Design review of the part built by this model. Coordinates are the model's own, in mm. A direction names the side the tool comes from. Coordinates: 2 decimals unless noted, no trailing zeros. Loops run counter-clockwise (first coordinate to the right, second up) from the corner with the lowest first, then second, coordinate; pieces in that order, holes last. Notation, with made-up numbers: (65.25, 86.25) -> (108.25, 86.25) arc R13 cw to (108.25, 105.25) -> close; hole circle Ø2 at (-1, 66.5). An arc over 180 degrees is marked (long way). Use one line per item in the form item = value. Start each with the question number.
1. Wall thickness on line 1 (Z direction, x = 82.5, y = 15); line 2 (Y direction, x = -37, z = 8.5); line 3 (X direction, y = 1, z = 25.5): over which ranges is each line inside the solid? List them lowest first. Write a range as from..to.
2. Consider section A-A (x = 32.5). State the section outline as (y, z) points, then the cut area to 3 significant figures.
3. Machinability: for faces 1 (the face through (1, 6, 25)), 2 (the face through (-72, 12, 25)), 3 (the face through (-30.699, 0.986, 27.825)), 4 (the face through (-25, 14, 25)), which of the approach directions +Z, -Z, +X, -X, +Y, -Y give a long, thin tool a straight path to every point of the face, cutting with its end or side? Answer none if there is none.
4. Consider section B-B (z = 42). State the section outline as (x, y) points, then the cut area to 3 significant figures.
5. Consider section C-C (x = -82.5). State the section outline as (y, z) points.
6. For pin 1 (15 mm diameter, centred on x = 10, z = 32, fed in from +Y); pin 2 (3 mm diameter, centred on x = -82.5, z = 8, fed in from -Y); pin 3 (0.6 mm diameter, centred on y = 1, z = 28, fed in from +X); pin 4 (1.5 mm diameter, centred on y = 8, z = 32.5, fed in from +X), all flat-tipped, find the tip position at first contact; note any pin that passes through.
7. Consider section D-D (z = 25). State how many separate pieces and enclosed holes the cut face has, then the cut area to 3 significant figures.
8. The part is to be moulded in two halves that separate along Y. For faces 5 (the face through (38.5, 4, 25)), 6 (the face through (1, 10, 50)), 7 (the face through (37, 0, 25)), say which applies: released by +Y, released by -Y, zero draft, split by the parting line, or undercut.
from build123d import *

# Parameters (mm, degrees)
SKETCH001_AS_DRAWN_R                 = 1.75
SKETCH001_AS_DRAWN_R_2               = 2.6
EXTRUDE003_DEPTH                     = 25
EXTRUDE003_ONTO_SKETCH001_ROLL_ANGLE = 90
SKETCH002_AS_DRAWN_R                 = 3.35
EXTRUDE002_DEPTH                     = 3
EXTRUDE002_ONTO_SKETCH002_ROLL_ANGLE = 90
EXTRUDE_DEPTH                        = 50


with BuildPart() as extrude003:
    # Sketch001 as drawn → Extrude003 (new)
    with BuildSketch(Plane.XY):
        with Locations((-82.5, -17)):
            Circle(SKETCH001_AS_DRAWN_R)
        with Locations((82.5, 17)):
            Circle(SKETCH001_AS_DRAWN_R)
        with Locations((82.5, -17)):
            Circle(SKETCH001_AS_DRAWN_R)
        with Locations((-32.5, 0)):
            Circle(SKETCH001_AS_DRAWN_R_2)
        with Locations((32.5, 0)):
            Circle(SKETCH001_AS_DRAWN_R_2)
        with Locations((-82.5, 17)):
            Circle(SKETCH001_AS_DRAWN_R)
    extrude(amount=-EXTRUDE003_DEPTH)


with BuildPart() as extrude003_1:
    # Extrude003 onto Sketch001 roll: moved
    add(extrude003.part.rotate(Axis((0, 0, 0), (1, 0, 0)), EXTRUDE003_ONTO_SKETCH001_ROLL_ANGLE))


with BuildPart() as extrude003_2:
    # Extrude003 onto Sketch001 placement: moved
    add(extrude003_1.part.moved(Location((0, 0, 25))))


with BuildPart() as fusion:
    # Sketch002 as drawn → Extrude002 (new)
    with BuildSketch(Plane.XY):
        with Locations((-32.5, 0)):
            Circle(SKETCH002_AS_DRAWN_R)
        with Locations((32.5, 0)):
            Circle(SKETCH002_AS_DRAWN_R)
    extrude(amount=-EXTRUDE002_DEPTH)


with BuildPart() as fusion_1:
    # Extrude002 onto Sketch002 roll: moved
    add(fusion.part.rotate(Axis((0, 0, 0), (1, 0, 0)), EXTRUDE002_ONTO_SKETCH002_ROLL_ANGLE))


with BuildPart() as fusion_2:
    # Extrude002 onto Sketch002 placement: moved
    add(fusion_1.part.moved(Location((0, 0, 25))))

    # Fusion: union Extrude003
    add(extrude003_2.part)


with BuildPart() as cut:
    # Sketch → Extrude (new body)
    with BuildSketch(Plane.XY):
        Polygon((90, 16), (90, 12), (55, 12), (45, 0), (25, 0), (25, 2), (38.5, 2), (38.5, 6), (-38.5, 6), (-38.5, 2), (-25, 2), (-25, 0), (-45, 0), (-55, 12), (-90, 12), (-90, 16), (-25, 16), (-25, 12), (25, 12), (25, 16), align=None)
    extrude(amount=EXTRUDE_DEPTH)

    # Cut: cut Fusion
    add(fusion_2.part, mode=Mode.SUBTRACT)


solid = cut.part
Geometry check:
q1.line_1 = 0..6.25, 9.75..40.25, 43.75..50
q1.line_2 = 0..2, 6..16
q1.line_3 = -45.83..-35.81, -29.19..-25, 25..29.19, 35.81..45.83
q2.outline = (0, 0) -> (2, 0) -> (2, 21.65) -> (0, 21.65) -> close; (0, 28.35) -> (2, 28.35) -> (2, 50) -> (0, 50) -> close; (6, 0) -> (16, 0) -> (16, 22.4) -> (6, 22.4) -> close; (6, 27.6) -> (16, 27.6) -> (16, 50) -> (6, 50) -> close
q2.area = 535 mm²
q3.face_1 = +Z, -Z
q3.face_2 = +Z, -Z, -X, -Y
q3.face_3 = -Y
q3.face_4 = +Z, -Z, +Y
q4.outline = (-90, 12) -> (-84.25, 12) -> (-84.25, 16) -> (-90, 16) -> close; (-80.75, 12) -> (-55, 12) -> (-45, 0) -> (-25, 0) -> (-25, 2) -> (-38.5, 2) -> (-38.5, 6) -> (38.5, 6) -> (38.5, 2) -> (25, 2) -> (25, 0) -> (45, 0) -> (55, 12) -> (80.75, 12) -> (80.75, 16) -> (25, 16) -> (25, 12) -> (-25, 12) -> (-25, 16) -> (-80.75, 16) -> close; (84.25, 12) -> (90, 12) -> (90, 16) -> (84.25, 16) -> close
q4.area = 1,280 mm²
q5.outline = (12, 0) -> (16, 0) -> (16, 6.25) -> (12, 6.25) -> close; (12, 9.75) -> (16, 9.75) -> (16, 40.25) -> (12, 40.25) -> close; (12, 43.75) -> (16, 43.75) -> (16, 50) -> (12, 50) -> close
q6.pin_1 = 12
q6.pin_2 = through
q6.pin_3 = 46.08
q6.pin_4 = 52.29
q7.separate_pieces = 5
q7.enclosed_holes = 0
q7.area = 1,180 mm²
q8.face_5 = undercut
q8.face_6 = zero draft
q8.face_7 = released by -Y
